For this review, take the finished solid that the model builds, in its own axes (mm). Give positions to 0.01 mm unless a question says otherwise; leave off trailing zeros. Loops run counter-clockwise (first coordinate to the right, second up) from the corner with the lowest first, then second, coordinate; pieces in that order, holes last. Notation, with made-up numbers: (48.5, 40) - (76.5, 40) arc R30 ccw to (76.5, 68) - close; hole circle Ø8 at (78, -19.5). An arc over 180 degrees is marked (long way). Answer in a Markdown table with one row per item.
```python
from build123d import *

# Parameters (mm, degrees)
SKETCH1_R           = 2.667
SKETCH1_R_2         = 1.905
SKETCH1_R_3         = 4.025
SKETCH1_R_4         = 2.032
BOSS_EXTRUDE1_DEPTH = 3.175


with BuildPart() as part:
    # Sketch1 → Boss-Extrude1 (new body)
    with BuildSketch(Plane(origin=(0, 0, 0), x_dir=(-1, 0, 0), z_dir=(0, 0, -1))):
        Polygon((2.749630657, 29.57498078), (-2.749630657, 29.57498078), (-24.237869343, 17.16874039), (-26.9875, 12.40624039), (-26.9875, -12.40624039), (-24.237869343, -17.16874039), (-2.749630657, -29.57498078), (2.749630657, -29.57498078), (24.237869343, -17.16874039), (26.9875, -12.40624039), (26.9875, 12.40624039), (24.237869343, 17.16874039), align=None)
        with Locations((20.622229928, 11.90625)):
            Circle(SKETCH1_R, mode=Mode.SUBTRACT)
        with Locations((0, -23.8125)):
            Circle(SKETCH1_R, mode=Mode.SUBTRACT)
        with Locations((-20.622229928, 11.90625)):
            Circle(SKETCH1_R, mode=Mode.SUBTRACT)
        with Locations((0, -8)):
            Circle(SKETCH1_R_2, mode=Mode.SUBTRACT)
        with Locations((0, 8)):
            Circle(SKETCH1_R_2, mode=Mode.SUBTRACT)
        with Locations((0, 23.8125)):
            Circle(SKETCH1_R, mode=Mode.SUBTRACT)
        Circle(SKETCH1_R_3, mode=Mode.SUBTRACT)
        with Locations((-8, 0)):
            Circle(SKETCH1_R_2, mode=Mode.SUBTRACT)
        with Locations((8, 0)):
            Circle(SKETCH1_R_2, mode=Mode.SUBTRACT)
        with Locations((-20.622229928, -11.90625)):
            Circle(SKETCH1_R, mode=Mode.SUBTRACT)
        with Locations((20.622229928, -11.90625)):
            Circle(SKETCH1_R, mode=Mode.SUBTRACT)
        with Locations((-6.914797213, 6.914797213)):
            Circle(SKETCH1_R_4, mode=Mode.SUBTRACT)
        with Locations((-6.914797213, -6.914797213)):
            Circle(SKETCH1_R_4, mode=Mode.SUBTRACT)
        with Locations((6.914797213, -6.914797213)):
            Circle(SKETCH1_R_4, mode=Mode.SUBTRACT)
        with Locations((6.914797213, 6.914797213)):
            Circle(SKETCH1_R_4, mode=Mode.SUBTRACT)
    extrude(amount=-BOSS_EXTRUDE1_DEPTH)


solid = part.part
```
1. Clearance check with flat-ended pins moving along their axes: pin 1 (2.5 mm diameter, centred on x = 8, y = 0, fed in from +Z) (3 decimals); pin 2 (1 mm diameter, centred on x = 18, z = 1.5, fed in from -Y). State where each tip first meets the part, or that it passes through.
Values:
| item | result |
|---|---|
| pin 1 | passes through |
| pin 2 | stops at y = -21.06 |
2. Wall thickness on line 1 (Y direction, x = -19.5, z = 2.35); line 2 (X direction, y = 6.5, z = 0.9); line 3 (X direction, y = 3, z = 2.1): over which ranges is each line inside the solid? List them lowest first. Write a range as [from, to].
Values:
| item | result |
|---|---|
| line 1 | y = [-19.9, -14.33], [-9.49, 9.49], [14.33, 19.9] |
| line 2 | x = [-26.99, -8.9], [-4.93, -1.17], [1.17, 4.93], [8.9, 26.99] |
| line 3 | x = [-26.99, -2.68], [2.68, 26.99] |
3. We need section A-A, the plane x = 0. Give the boundary of the cut face in (y, z) (1 decimal).
Values:
| item | result |
|---|---|
| outline | (-29.6, 0) - (-26.5, 0) - (-26.5, 3.2) - (-29.6, 3.2) - close; (-21.1, 0) - (-9.9, 0) - (-9.9, 3.2) - (-21.1, 3.2) - close; (-6.1, 0) - (-4, 0) - (-4, 3.2) - (-6.1, 3.2) - close; (4, 0) - (6.1, 0) - (6.1, 3.2) - (4, 3.2) - close; (9.9, 0) - (21.1, 0) - (21.1, 3.2) - (9.9, 3.2) - close; (26.5, 0) - (29.6, 0) - (29.6, 3.2) - (26.5, 3.2) - close |
4. Mouldability with a two-part tool opening along Y and no side actions: class faces 1 (the face through (0.25, -6.11, 1.57)), 2 (the face through (-13.644, 23.285, 1.565)), 3 (the face through (25.632, -14.754, 1.565)) as released by +Y, released by -Y, zero draft, split by the parting line, or undercut.
Values:
| item | result |
|---|---|
| face 1 | undercut |
| face 2 | released by +Y |
| face 3 | released by -Y |
5. We need section B-B, the plane y = 22.5. Give the boundary of the cut face in (x, z) (3 decimals), and give its area (3 significant figures).
Values:
| item | result |
|---|---|
| outline | (-15.004, 0) - (-2.322, 0) - (-2.322, 3.175) - (-15.004, 3.175) - close; (2.322, 0) - (15.004, 0) - (15.004, 3.175) - (2.322, 3.175) - close |
| area | 80.5 mm^2 |
6. We need section D-D, the plane x = -8. Give the boundary of the cut face in (y, z) (3 decimals).
Values:
| item | result |
|---|---|
| outline | (-26.544, 0) - (-8.633, 0) - (-8.633, 3.175) - (-26.544, 3.175) - close; (-5.197, 0) - (-1.905, 0) - (-1.905, 3.175) - (-5.197, 3.175) - close; (1.905, 0) - (5.197, 0) - (5.197, 3.175) - (1.905, 3.175) - close; (8.633, 0) - (26.544, 0) - (26.544, 3.175) - (8.633, 3.175) - close |
7. We need section C-C, the plane y = -1. Give the boundary of the cut face in (x, z) (1 decimal).
Values:
| item | result |
|---|---|
| outline | (-27, 0) - (-9.6, 0) - (-9.6, 3.2) - (-27, 3.2) - close; (-6.4, 0) - (-3.9, 0) - (-3.9, 3.2) - (-6.4, 3.2) - close; (3.9, 0) - (6.4, 0) - (6.4, 3.2) - (3.9, 3.2) - close; (9.6, 0) - (27, 0) - (27, 3.2) - (9.6, 3.2) - close |
